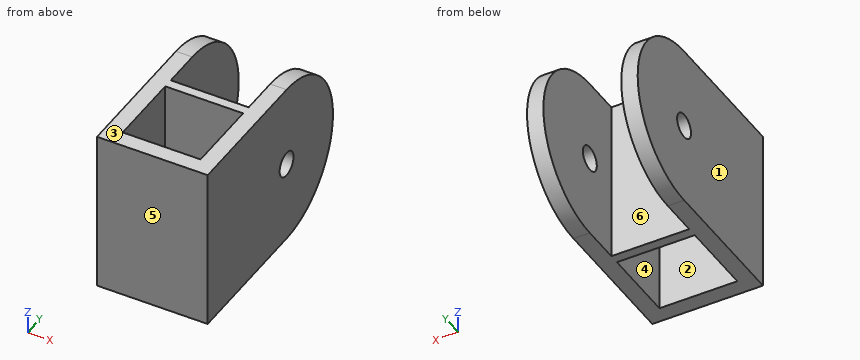
Autodesk Inventor part; units mm, degrees
ref_plane "YZ Plane" through (0, 0, 0) normal (1, 0, 0) x (0, 1, 0)
ref_plane "XZ Plane" through (0, 0, 0) normal (0, 1, 0) x (-1, 0, 0)
ref_plane "XY Plane" through (0, 0, 0) normal (0, 0, 1) x (1, 0, 0)
sketch "Boceto1" plane through (0, 0, 0) normal (0, 1, 0) x (-1, 0, 0)
  line L0 (0, 0) -> (27, 0)
  line L1 (27, 0) -> (27, -40)
  line L2 (27, -40) -> (0, -40)
  line L3 (0, -40) -> (0, 0)
  dimension "d0" = 27
  dimension "d1" = 40
extrude "Extrusión1" add sketch "Boceto1" along normal blind 54
sketch "Boceto2" plane through (-27, 0, 0) normal (0, 0, 1) x (1, 0, 0)
  line L0 (4, 4) -> (23, 4)
  line L1 (23, 4) -> (23, 22.3365)
  line L2 (23, 22.3365) -> (4, 22.3365)
  line L3 (4, 22.3365) -> (4, 4)
  line L4 (0, 0) -> (27, 0)
  line L5 (27, 0) -> (27, 54)
  line L6 (0, 54) -> (27, 54)
  line L7 (0, 0) -> (0, 54)
  line L8 (27, 54) -> (0, 54)
  line L9 (4, 24.7292) -> (23, 24.7292)
  line L10 (23, 24.7292) -> (23, 54)
  line L11 (23, 54) -> (4, 54)
  line L12 (4, 54) -> (4, 24.7292)
  point P0 (4, 54)
  dimension "d4" = 4
  dimension "d5" = 4
  dimension "d6" = 4
extrude "Extrusión2" cut sketch "Boceto2" against normal blind 54 contours L3 L2 L1 L0 | L6 L10 L9 L12
sketch "Boceto3" plane through (0, 0, 0) normal (1, 0, 0) x (0, 0, -1)
  line L0 (0, 0) -> (40, 0)
  line L1 (40, 0) -> (40, 54)
  line L2 (0, 54) -> (40, 54)
  line L3 (0, 0) -> (0, 54)
  line L4 (0, 54) -> (40, 54)
  line L5 (20, 54) -> (20, 34)
  circle A0 centre (20, 34) radius 3
  dimension "d9" = 20
  dimension "d10" = 6
extrude "Extrusión3" cut sketch "Boceto3" against normal blind 54 contours A0
sketch "Boceto4" plane through (0, 0, 0) normal (1, 0, 0) x (0, 0, -1)
  circle A0 centre (20, 34) radius 3
  line L0 (0, 0) -> (40, 0)
  line L1 (40, 0) -> (40, 54)
  line L2 (0, 54) -> (40, 54)
  line L3 (0, 0) -> (0, 54)
  line L4 (40, 54) -> (0, 54)
  circle A1 centre (20, 34) radius 3
  circle A2 centre (20, 34) radius 20
  point P0 (0, 34)
  point P1 (20, 54)
  point P2 (40, 34)
extrude "Extrusión4" cut sketch "Boceto4" against normal blind 54 contours L3 L2 A2 | A2 L2 L1
properties part number "REDONDA"
Part model, mm, in its own coordinate system. Face numbers are marked on the shaded views. A direction names the side the tool comes from. Give positions to 0.01 mm unless a question says otherwise; leave off trailing zeros. Loops run counter-clockwise (first coordinate to the right, second up) from the corner with the lowest first, then second, coordinate; pieces in that order, holes last.
(1) Pin check, flat tips, straight feed: pin 1 (8 mm diameter, centred on x = -18, z = -34, fed in from +Y); pin 2 (10 mm diameter, centred on x = -21, z = -17, fed in from +Y); pin 3 (12 mm diameter, centred on x = -22, z = -9, fed in from +Y). Stop position of each tip, or through.
Return value:
pin 1: stops at y = 24.73
pin 2: stops at y = 54
pin 3: stops at y = 53.34
(2) Band-saw the part on A-A (z = -20). Write the cut outline in (x, y), and give its area (3 significant figures).
Return value:
outline: (-27, 0) - (0, 0) - (0, 31) - (-4, 31) - (-4, 24.73) - (-23, 24.73) - (-23, 31) - (-27, 31) - close; (-27, 37) - (-23, 37) - (-23, 54) - (-27, 54) - close; (-4, 37) - (0, 37) - (0, 54) - (-4, 54) - close; hole (-23, 4) - (-4, 4) - (-4, 22.34) - (-23, 22.34) - close
area: 505 mm2
(3) Pull direction X, two halves, no side cores. Call the marked faces 1, 2 and 3: pulls with the +X half, pulls with the -X half, needs draft (parallel to the pull), parting line crosses it, or undercut.
Return value:
face 1: pulls with the -X half
face 2: undercut
face 3: needs draft
(4) Drill centre lines: line 1 along Y through (x, z) = (-16, -37); line 2 along X through (y, z) = (35, -15); line 3 along Y through (x, z) = (-2.6, -20). Where is each one in solid material? Low to high.
Return value:
line 1: y = 0 to 4, 22.34 to 24.73
line 2: x = -27 to -23, -4 to 0
line 3: y = 0 to 31, 37 to 54
(5) 3-axis set-ups, long thin cutter, end or side, ignore diameter. For the marked faces 4, 5 and 6: which of +Z, -Z, +X, -X, +Y, -Y reach the whole face in a straight line?
Return value:
face 4: +Z, -Z
face 5: +Z, -Z, +X, -X, -Y
face 6: +Z, -Z, +Y
(6) Band-saw the part on D-D (z = -31). Write the cut outline in (x, y), and give its area (3 significant figures).
Return value:
outline: (-27, 0) - (0, 0) - (0, 50.7) - (-4, 50.7) - (-4, 24.73) - (-23, 24.73) - (-23, 50.7) - (-27, 50.7) - close; hole (-23, 4) - (-4, 4) - (-4, 22.34) - (-23, 22.34) - close
area: 527 mm2
(7) Band-saw the part on C-C (x = -5). Write the cut outline in (y, z), and give its area (3 significant figures).
Return value:
outline: (0, -40) - (4, -40) - (4, 0) - (0, 0) - close; (22.34, -40) - (24.73, -40) - (24.73, 0) - (22.34, 0) - close
area: 256 mm2
(8) Band-saw the part on B-B (y = 11). Write the cut outline in (x, z), and give its area (3 significant figures).
Return value:
outline: (-27, -40) - (-23, -40) - (-23, 0) - (-27, 0) - close; (-4, -40) - (0, -40) - (0, 0) - (-4, 0) - close
area: 320 mm2
